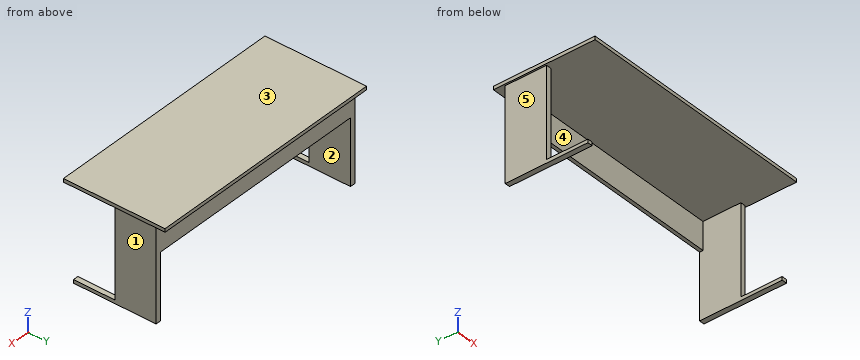
```python
from build123d import *

# Parameters (mm, degrees)
F0_W     = 1778
F0_H     = 749.3
F1_DEPTH = 25.4
F2_W     = 38.1
F2_H     = 304.8
F3_DEPTH = 660.4
F5_W     = 38.1
F5_H     = 609.6
F4_W     = 38.1
F4_H     = 609.6
F6_DEPTH = 25.4
F7_W     = 25.4
F7_H     = 203.2
F8_DEPTH = 1676.4


with BuildPart() as f1:
    # F0 (on Top) → F1 (new body)
    with BuildSketch(Plane.XY):
        Rectangle(F0_W, F0_H)
    extrude(amount=-F1_DEPTH)

    # F2 (on face) → F3 (join)
    with BuildSketch(Plane(origin=(0, 0, -25.4), x_dir=(1, 0, 0), z_dir=(0, 0, -1))):
        with Locations((857.25, -146.05)):
            Rectangle(F2_W, F2_H)
        with Locations((-857.25, -146.05)):
            Rectangle(F2_W, F2_H)
    extrude(amount=F3_DEPTH)

    # F5 (on face) + F4 (on face) → F6 (join)
    with BuildSketch(Plane(origin=(0, 0, -685.8), x_dir=(1, 0, 0), z_dir=(0, 0, -1))):
        with Locations((-857.25, 6.35)):
            Rectangle(F5_W, F5_H)
    with BuildSketch(Plane(origin=(0, 0, -685.8), x_dir=(1, 0, 0), z_dir=(0, 0, -1))):
        with Locations((857.25, 6.35)):
            Rectangle(F4_W, F4_H)
    extrude(amount=F6_DEPTH)

    # F7 (on face) → F8 (join, through all)
    with BuildSketch(Plane.YZ.offset(-838.2)):
        with Locations((285.75, -127)):
            Rectangle(F7_W, F7_H)
    extrude(amount=F8_DEPTH)


solid = f1.part
```
Work out the finished part from the listing and answer in its coordinate system (mm). Face numbers are marked on the shaded views. A direction names the side the tool comes from. Coordinates: 2 decimals unless noted, no trailing zeros. Loops run counter-clockwise (first coordinate to the right, second up) from the corner with the lowest first, then second, coordinate; pieces in that order, holes last. Notation, with made-up numbers: M 29.5,64 L 86.5,64 A30 cw 86.5,88 Z; hole C -26.5,-16.75 d10. An arc over 180 degrees is marked long. Use CSV: the item, a comma, the result in double quotes. Start each with the question number.
(1) For the marked faces 4 and 5, determine the directions among +Z, -Z, +X, -X, +Y, -Y from which every point of the face is accessible in a straight line to the end or side of a thin tool.
(2) Find section C-C, the plane x = 579.5. Give the vertices of the cut face in (y, z), then the cut area to 3 significant figures.
(3) Find section B-B, the plane y = -266. Give the vertices of the cut face in (x, z), then the cut area to 3 significant figures.
(4) Given pin 1 Ø11.5 at (x, z) = (-865, -415.5) entering from -Y; pin 2 Ø20.5 at (x, z) = (-850.5, -697) entering from -Y; pin 3 Ø1 at (y, z) = (30, -310.5) entering from +X, each flat-ended and moving along its own axis, determine where each tip first touches the part or whether it passes through.
(5) For a pull along X with two mould halves and no side action, classify the marked faces 1, 2 and 3 as +X half, -X half, draft (parallel to the pull), parting line (faces both ways), or undercut.
(6) Consider line 1 (X direction, y = 190, z = -114.5); line 2 (Y direction, x = 247.5, z = -110.5). Determine where each line is inside the solid, lowest interval first.
(7) Find section D-D, the plane z = -52. Give the vertices of the cut face in (x, y), then the cut area to 3 significant figures.
(8) Find section A-A, the plane z = -490. Give the vertices of the cut face in (x, y).
Recorded:
1,face 4,"-Z, -Y"
1,face 5,"-Z, -X, +Y, -Y"
2,outline,"M -374.65,-25.4 L 273.05,-25.4 L 273.05,-228.6 L 298.45,-228.6 L 298.45,-25.4 L 374.65,-25.4 L 374.65,0 L -374.65,0 Z"
2,area,"24,200 mm^2"
3,outline,"M -889,-25.4 L 889,-25.4 L 889,0 L -889,0 Z; M -876.3,-711.2 L -838.2,-711.2 L -838.2,-685.8 L -876.3,-685.8 Z; M 838.2,-711.2 L 876.3,-711.2 L 876.3,-685.8 L 838.2,-685.8 Z"
3,area,"47,100 mm^2"
4,pin 1,"stops at y = -6.35"
4,pin 2,"stops at y = -311.15"
4,pin 3,"stops at x = 876.3"
5,face 1,"+X half"
5,face 2,"undercut"
5,face 3,"draft"
6,line 1,"x = -876.3 to -838.2, 838.2 to 876.3"
6,line 2,"y = 273.05 to 298.45"
7,outline,"M -876.3,-6.35 L -838.2,-6.35 L -838.2,273.05 L 838.2,273.05 L 838.2,-6.35 L 876.3,-6.35 L 876.3,298.45 L -876.3,298.45 Z"
7,area,"65,800 mm^2"
8,outline,"M -876.3,-6.35 L -838.2,-6.35 L -838.2,298.45 L -876.3,298.45 Z; M 838.2,-6.35 L 876.3,-6.35 L 876.3,298.45 L 838.2,298.45 Z"
